Geometry: final body of the model. Coordinates: model frame, mm. A direction names the side the tool comes from. Coordinates: 2 decimals unless noted, no trailing zeros. Order: outer loops, then holes, each group sorted by start corner. A loop starts at its lowest first (then second) coordinate and runs counter-clockwise, first axis right, second up. Notation, with made-up numbers: (9, -21.5) -> (55, -21.5) arc R6 cw to (55, -14.5) -> close; hole circle Ø9 at (70.5, 22). An arc over 180 degrees is marked (long way). Use CSV: the item, a comma, the result in double quotes. Start each with the question number.
from build123d import *

# Parameters (mm, degrees)
SKETCH1_W                     = 52.5
SKETCH1_H                     = 35.73
BOSS_EXTRUDE1_DEPTH           = 10
SKETCH3_R                     = 1.5
CUT_EXTRUDE1_DEPTH            = 10
CBORE_FOR_M4_SHCS1_AT_2_COUNT = 2
CBORE_FOR_M4_SHCS1_AT_2_PITCH = 24


with BuildPart() as part:
    # Sketch1 → Boss-Extrude1 (new body)
    with BuildSketch(Plane(origin=(0, 0, 0), x_dir=(1, 0, 0), z_dir=(0, 1, 0))):
        with Locations((26.25, 17.865)):
            Rectangle(SKETCH1_W, SKETCH1_H)
    extrude(amount=BOSS_EXTRUDE1_DEPTH)

    # Sketch3 → Cut-Extrude1 (cut)
    with BuildSketch(Plane.ZY):
        with Locations((-27.865, 5)):
            Circle(SKETCH3_R)
        with Locations((-7.865, 5)):
            Circle(SKETCH3_R)
    cut_extrude1 = extrude(amount=-CUT_EXTRUDE1_DEPTH, mode=Mode.SUBTRACT)

    # Mirror1: Cut-Extrude1 across plane
    add(cut_extrude1.mirror(Plane(origin=(26.25, 0, 0), x_dir=(0, 0, 1), z_dir=(1, 0, 0))), mode=Mode.SUBTRACT)

    # Sketch6 → CBORE for M4 SHCS1 (revolve, cut)
    with BuildSketch(Plane(origin=(38.25, 10, -17.865), x_dir=(0, 0, 1), z_dir=(1, 0, 0))):
        Polygon((0, 0), (0, 10), (2.25, 10), (2.25, 4), (4, 4), (4, 0.025), (4.025, 0), align=None)
    cbore_for_m4_shcs1 = revolve(axis=Axis((38.25, 16.35, -17.865), (0, -1, 0)), mode=Mode.SUBTRACT)

    # CBORE for M4 SHCS1 at 2: CBORE for M4 SHCS1 ×2
    with Locations(*[(-i * CBORE_FOR_M4_SHCS1_AT_2_PITCH, 0, 0) for i in range(1, CBORE_FOR_M4_SHCS1_AT_2_COUNT)]):
        add(cbore_for_m4_shcs1, mode=Mode.SUBTRACT)


solid = part.part
(1) Line query: line 1 (Z direction, x = 2, y = 5.5); line 2 (Z direction, x = 38.25, y = 3.7) (3 decimals); line 3 (Z direction, x = 17, y = 6.75). Output: solid intervals per line, ascending. Write a range as from..to.
(2) Section C-C (z = -7.5). Return loops of the section in (x, y).
(3) First-contact query: pin 1 (2.5 mm diameter, centred on y = 5, z = -7.865, fed in from -X); pin 2 (4 mm diameter, centred on x = 37.5, z = -18, fed in from +Y); pin 3 (0.9 mm diameter, centred on y = 4.5, z = -7, fed in from +X). Flat tips, straight axial feed; report the tip coordinate or a pass-through.
(4) Section D-D (z = -19). State how many separate pieces and enclosed holes the cut face has, then the cut area to 3 significant figures.
(5) Section B-B (y = 5). Return loops of the section in (x, z) (3 decimals), then the cut area to 3 significant figures.
(6) Access query for faces 1 (the face through (42.5, 5, -8)), 2 (the face through (4.93, 5.066, -9.364)), 3 (the face through (40, 6, -20)). Directions: +Z, -Z, +X, -X, +Y, -Y. A direction counts if a zero-diameter tool reaches every point of the face in a straight line with its end or side. Return the directions, or none.
(7) Section A-A (x = 14.25). Return loops of the section in (y, z) (3 decimals), then the cut area to 3 significant figures.
(8) Mould query, pull axis X, two halves, no side actions, for faces 4 (the face through (26, 5, 0)), 5 (the face through (16.25, 3.04, -16.83)), 6 (the face through (0, 5, -18)), 7 (the face through (34.88, 8.02, -15.71)). Classes: pulls with the +X half, pulls with the -X half, needs draft (parallel to the pull), parting line crosses it, or undercut.
Check sheet entries:
1,line 1,"z = -35.73..-29.28, -26.45..-9.28, -6.45..0"
1,line 2,"z = -35.73..-20.115, -15.615..0"
1,line 3,"z = -35.73..-20.77, -14.96..0"
2,outline,"(0, 0) -> (52.5, 0) -> (52.5, 3.55) -> (42.5, 3.55) -> (42.5, 6.45) -> (52.5, 6.45) -> (52.5, 10) -> (0, 10) -> (0, 6.45) -> (10, 6.45) -> (10, 3.55) -> (0, 3.55) -> close"
3,pin 1,"stops at x = 10"
3,pin 2,"stops at y = 6"
3,pin 3,"stops at x = 42.5"
4,separate pieces,"3"
4,enclosed holes,"0"
4,area,"417 mm^2"
5,outline,"(0, -35.73) -> (52.5, -35.73) -> (52.5, -29.365) -> (42.5, -29.365) -> (42.5, -26.365) -> (52.5, -26.365) -> (52.5, -9.365) -> (42.5, -9.365) -> (42.5, -6.365) -> (52.5, -6.365) -> (52.5, 0) -> (0, 0) -> (0, -6.365) -> (10, -6.365) -> (10, -9.365) -> (0, -9.365) -> (0, -26.365) -> (10, -26.365) -> (10, -29.365) -> (0, -29.365) -> close; hole circle Ø4.5 at (14.25, -17.865); hole circle Ø4.5 at (38.25, -17.865)"
5,area,"1,720 mm^2"
6,face 1,"+X"
6,face 2,"-X"
6,face 3,"+Y"
7,outline,"(0, -35.73) -> (10, -35.73) -> (10, -21.89) -> (9.975, -21.865) -> (6, -21.865) -> (6, -20.115) -> (0, -20.115) -> close; (0, -15.615) -> (6, -15.615) -> (6, -13.865) -> (9.975, -13.865) -> (10, -13.84) -> (10, 0) -> (0, 0) -> close"
7,area,"298 mm^2"
8,face 4,"needs draft"
8,face 5,"undercut"
8,face 6,"pulls with the -X half"
8,face 7,"undercut"
